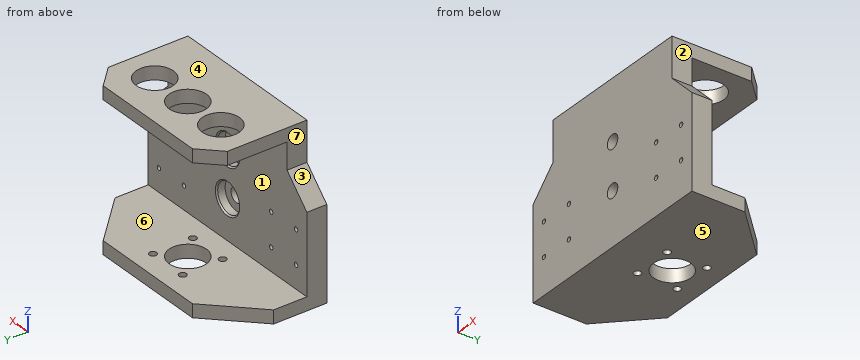
```python
from build123d import *

# Parameters (mm, degrees)
SKETCH1_W                                    = 101.6
SKETCH1_H                                    = 76.2
BOSS_EXTRUDE1_DEPTH                          = 50.8
CUT_EXTRUDE1_DEPTH                           = 31.75
CUT_EXTRUDE1_DEPTH_BACK                      = 31.75
SKETCH9_W                                    = 101.6
SKETCH9_H                                    = 41.275
F_45_64_0_70313_DIAMETER_HOLE1_D             = 17.859502
F_45_64_0_70313_DIAMETER_HOLE2_D             = 17.859502
F_45_64_0_70313_DIAMETER_HOLE2_DEPTH         = 25.4
F_45_64_0_70313_DIAMETER_HOLE2_TIP           = 5.365535714
CBORE_FOR_1_4_BINDING_HEAD_MACHINE_S_2_COUNT = 2
CBORE_FOR_1_4_BINDING_HEAD_MACHINE_S_2_PITCH = 22.098
CUT_EXTRUDE3_DEPTH                           = 137.783186101
F_8_32_TAPPED_HOLE1_D                        = 3.4544
F_8_32_TAPPED_HOLE1_DEPTH                    = 6.35
CUT_EXTRUDE4_DEPTH                           = 136.636059457
F_44_0_086_DIAMETER_HOLE1_D                  = 2.1844


with BuildPart() as part:
    # Sketch1 → Boss-Extrude1 (new body)
    with BuildSketch(Plane(origin=(0, 0, 0), x_dir=(1, 0, 0), z_dir=(0, 1, 0))):
        with Locations((50.8, 38.1)):
            Rectangle(SKETCH1_W, SKETCH1_H)
    extrude(amount=BOSS_EXTRUDE1_DEPTH)

    # Sketch9 → Cut-Extrude1 (cut, two sides: drawn at the far end of the back side and taken through both)
    with BuildSketch(Plane.XY.offset(-38.1).offset(-CUT_EXTRUDE1_DEPTH_BACK)):
        with Locations((50.8, 30.1625)):
            Rectangle(SKETCH9_W, SKETCH9_H)
    extrude(amount=CUT_EXTRUDE1_DEPTH + CUT_EXTRUDE1_DEPTH_BACK, mode=Mode.SUBTRACT)

    # 45/64 (0.70313) Diameter Hole1 (through all)
    with Locations(Plane.XY):
        with Locations((50.8, 28.5242)):
            Hole(F_45_64_0_70313_DIAMETER_HOLE1_D / 2)

    # 45/64 (0.70313) Diameter Hole2
    with Locations(Plane.XY):
        with Locations((29.6418, 28.5242), (71.9582, 28.5242)):
            Hole(F_45_64_0_70313_DIAMETER_HOLE2_D / 2, depth=F_45_64_0_70313_DIAMETER_HOLE2_DEPTH)
            with Locations((0, 0, -(F_45_64_0_70313_DIAMETER_HOLE2_DEPTH + F_45_64_0_70313_DIAMETER_HOLE2_TIP / 2))):  # 118° drill point
                Cone(0, F_45_64_0_70313_DIAMETER_HOLE2_D / 2, F_45_64_0_70313_DIAMETER_HOLE2_TIP, mode=Mode.SUBTRACT)

    # Sketch14 → CBORE for 1/4 Binding Head Machine Screw1 (revolve, cut)
    with BuildSketch(Plane(origin=(50.8, 9.525, -50.8), x_dir=(0, 0, 1), z_dir=(1, 0, 0))):
        Polygon((0, 0), (0, 9.525), (3.3782, 9.525), (3.3782, 4.191), (7.14375, 4.191), (7.14375, 0.635), (7.77875, 0), align=None)
    cbore_for_1_4_binding_head_machine_screw = revolve(axis=Axis((50.8, 15.875, -50.8), (0, -1, 0)), mode=Mode.SUBTRACT)

    # CBORE for 1_4 Binding Head Machine S 2: CBORE for 1/4 Binding Head Machine Screw1 ×2
    with Locations(*[(0, 0, i * CBORE_FOR_1_4_BINDING_HEAD_MACHINE_S_2_PITCH) for i in range(1, CBORE_FOR_1_4_BINDING_HEAD_MACHINE_S_2_COUNT)]):
        add(cbore_for_1_4_binding_head_machine_screw, mode=Mode.SUBTRACT)

    # Sketch17 → Cut-Extrude3 (cut, through all)
    with BuildSketch(Plane.XY):
        Polygon((0, 25.4), (22.225, 47.625), (79.375, 47.625), (101.6, 25.4), (101.6, 50.8), (0, 50.8), align=None)
    extrude(amount=-CUT_EXTRUDE3_DEPTH, mode=Mode.SUBTRACT)

    # #8-32 Tapped Hole1
    with Locations(Plane(origin=(0, 0, -76.2), x_dir=(-1, 0, 0), z_dir=(0, 0, -1))):
        with Locations((-41.275, 38.0492), (-60.325, 18.9992), (-60.325, 38.0492), (-41.275, 18.9992)):
            Hole(F_8_32_TAPPED_HOLE1_D / 2, depth=F_8_32_TAPPED_HOLE1_DEPTH)

    # Sketch21 → Cut-Extrude4 (cut, through all)
    with BuildSketch(Plane.XZ):
        Polygon((0, 0), (0, -31.75), (12.7, -19.05), (12.7, 0), align=None)
        Polygon((88.9, 0), (101.6, 0), (101.6, -31.75), (88.9, -19.05), align=None)
    extrude(amount=-CUT_EXTRUDE4_DEPTH, mode=Mode.SUBTRACT)

    # #44 (0.086) Diameter Hole1 (through all)
    with Locations(Plane(origin=(0, 0, 0), x_dir=(-1, 0, 0), z_dir=(0, -1, 0))):
        with Locations((-22.8844, 58.8518), (-6.8844, 58.8518), (-22.8844, 42.8518), (-6.8844, 42.8518), (-78.7156, 58.8518), (-94.7156, 58.8518), (-78.7156, 42.8518), (-94.7156, 42.8518)):
            Hole(F_44_0_086_DIAMETER_HOLE1_D / 2)


solid = part.part
```
Work out the finished part from the listing and answer in its coordinate system (mm). Face numbers are marked on the shaded views. A direction names the side the tool comes from. Give positions to 0.01 mm unless a question says otherwise; leave off trailing zeros. Write each loop counter-clockwise with the first axis right and the second up, starting at its lowest first coordinate (ties: lowest second). Pieces come first, ordered by that corner, then holes. Notation, with made-up numbers: (88, 22.5) -> (106, 22.5) arc R15 cw to (106, 35.5) -> close; hole circle Ø2 at (-22, 56). An arc over 180 degrees is marked (long way). Write each question's results on one line, items separated by ' | '.
1. Each of these flat-tipped pins is pushed along its axis until it touches: pin 1 Ø21 at (y, z) = (19.5, -8.5) entering from +X; pin 2 Ø4 at (x, y) = (41.28, 19) entering from +Z; pin 3 Ø3 at (x, z) = (31, -60.5) entering from +Y (3 decimals); pin 4 Ø1.3 at (x, z) = (6.88, -58.85) entering from +Y. Where does it stop, or does it pass through?
Data:
pin 1: x = 88.9 | pin 2: z = 0 | pin 3: y = 9.525 | pin 4: through
2. Find section A-A on z = -50.8. Determine the outline of the cut face in (x, y) (3 decimals), and give its area (3 significant figures).
Data:
outline: (0, 0) -> (47.422, 0) -> (47.422, 5.334) -> (43.656, 5.334) -> (43.656, 8.89) -> (43.021, 9.525) -> (0, 9.525) -> close; (54.178, 0) -> (101.6, 0) -> (101.6, 9.525) -> (58.579, 9.525) -> (57.944, 8.89) -> (57.944, 5.334) -> (54.178, 5.334) -> close | area: 871 mm^2
3. Determine the mould class of the marked faces 4, 5, 6 and 7 for opening direction Z: +Z half, -Z half, draft (parallel to the pull), parting line (faces both ways), or undercut.
Data:
face 4: +Z half | face 5: -Z half | face 6: undercut | face 7: draft
4. A tool of negligible diameter and unlimited length cuts with its end or side. For the marked faces 1, 2 and 3, from which of +Z, -Z, +X, -X, +Y, -Y can it reach the whole face along a straight path? Write none if from no direction.
Data:
face 1: +X, -X, +Y | face 2: +Z, +X, +Y, -Y | face 3: +Z, -X, +Y, -Y
5. Straight lines are drawn through the part: L1, parallel to X at y = 19, z = -72.5; L2, parallel to Z at x = 67, y = 13; L3, parallel to Z at x = 91, y = 35. For each, find the intervals that lie inside material, in ascending order.
Data:
L1: 0 to 39.55, 43 to 58.6, 62.05 to 101.6 | L2: -76.2 to -69.85, -6.35 to 0 | L3: -76.2 to -69.85
6. Find section B-B on x = 50.8. Give the number of separate pieces and of enclosed holes in the cut face, and give its area (3 significant figures).
Data:
separate pieces: 5 | enclosed holes: 0 | area: 790 mm^2
7. Find section D-D on x = 27.5. Determine the outline of the cut face in (y, z) (3 decimals), and give its area (3 significant figures).
Data:
outline: (0, -76.2) -> (47.625, -76.2) -> (47.625, -69.85) -> (9.525, -69.85) -> (9.525, -6.35) -> (19.855, -6.35) -> (19.855, 0) -> (0, 0) -> close; (37.193, -6.35) -> (47.625, -6.35) -> (47.625, 0) -> (37.193, 0) -> close | area: 1,100 mm^2
8. Find section C-C on y = 27. Determine the outline of the cut face in (x, z), and give its area (3 significant figures).
Data:
outline: (1.6, -76.2) -> (42, -76.2) -> (42, -69.85) -> (1.6, -69.85) -> close; (12.7, -6.35) -> (20.84, -6.35) -> (20.84, 0) -> (12.7, 0) -> close; (38.44, -6.35) -> (42, -6.35) -> (42, 0) -> (38.44, 0) -> close; (59.6, -76.2) -> (100, -76.2) -> (100, -69.85) -> (59.6, -69.85) -> close; (59.6, -6.35) -> (63.16, -6.35) -> (63.16, 0) -> (59.6, 0) -> close; (80.76, -6.35) -> (88.9, -6.35) -> (88.9, 0) -> (80.76, 0) -> close | area: 662 mm^2
